Answer from the drawing. Dimensions are ordinates in mm from the lowest x, y and z of the part. Round coordinates to 2 decimals unless told otherwise and drop trailing zeros. Write each loop counter-clockwise with the first axis right and the second up, starting at its lowest first coordinate (ties: lowest second). Pieces come first, ordered by that corner, then holes. Notation, with made-up numbers: (87.25, 16) - (129.25, 16) arc R20 ccw to (129.25, 28) - close; hole circle Ø5 at (-1, 22). An arc over 180 degrees is marked (long way). One line per item, written item: value. Start each with the question number.
(1) A cutting plane is placed at D-D, the plane x = 8.25. Determine the outline of the cut face in (y, z), plus the area to 3 significant figures.
(2) Find the intervals of material crossed by L1, parallel to X at y = 0.15, z = 4; L2, parallel to Z at x = 13, y = 0.25; L3, parallel to Z at x = 2.5, y = 0.15, in increasing order.
(3) A cutting plane is placed at B-B, the plane x = 4. Determine the outline of the cut face in (y, z), plus the area to 3 significant figures.
(4) A cutting plane is placed at C-C, the plane z = 6.5. Determine the outline of the cut face in (x, y).
(5) A cutting plane is placed at A-A, the plane y = 0.2. Determine the outline of the cut face in (x, z), plus the area to 3 significant figures.
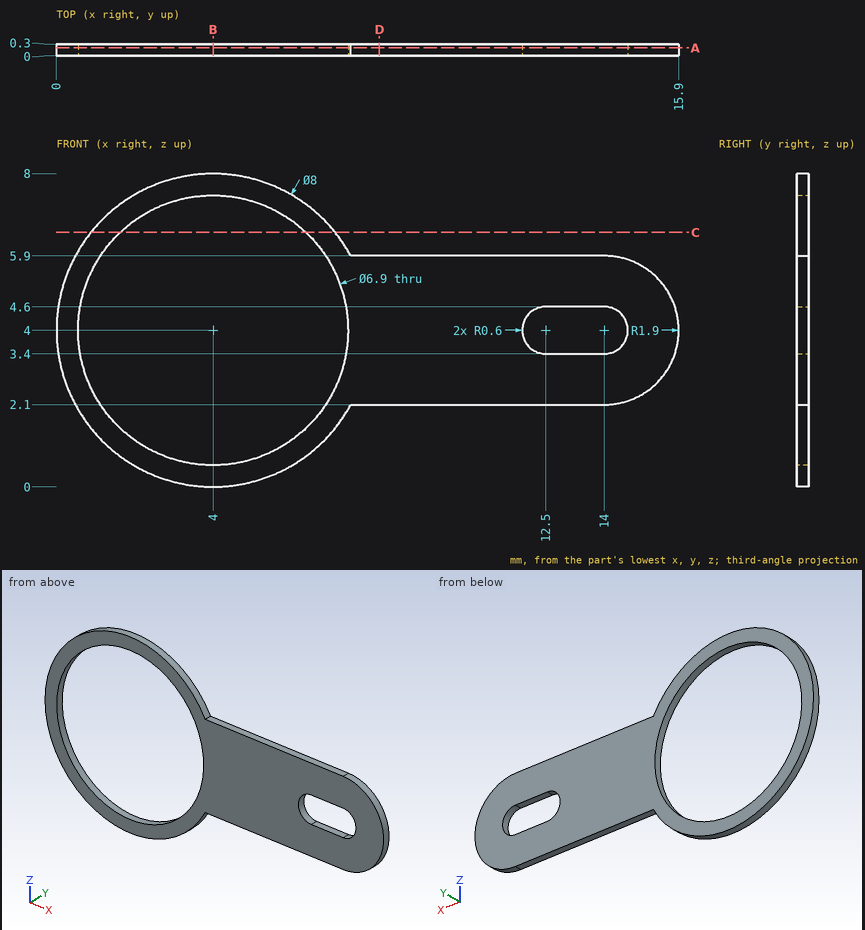
Here are the results:
1. outline: (0, 2.1) - (0.3, 2.1) - (0.3, 5.9) - (0, 5.9) - close
1. area: 1.14 mm²
2. L1: 0 to 0.55, 7.45 to 11.9, 14.6 to 15.9
2. L2: 2.1 to 3.4, 4.6 to 5.9
2. L3: 0.29 to 0.89, 7.11 to 7.71
3. outline: (0, 0) - (0.3, 0) - (0.3, 0.55) - (0, 0.55) - close; (0, 7.45) - (0.3, 7.45) - (0.3, 8) - (0, 8) - close
3. area: 0.330 mm²
4. outline: (0.88, 0) - (1.62, 0) - (1.62, 0.3) - (0.88, 0.3) - close; (6.38, 0) - (7.12, 0) - (7.12, 0.3) - (6.38, 0.3) - close
5. outline: (7.52, 2.1) - (14, 2.1) arc R1.9 ccw to (14, 5.9) - (7.52, 5.9) arc R4 ccw (long way) to start; hole circle Ø6.9 at (4, 4); hole (12.5, 3.4) - (14, 3.4) arc R0.6 ccw to (14, 4.6) - (12.5, 4.6) arc R0.6 ccw to start
5. area: 39.0 mm²
